from build123d import *

# Parameters (mm, degrees)
SKETCH1_W           = 20.32
SKETCH1_H           = 20.32
BOSS_EXTRUDE1_DEPTH = 1.905
CUT_EXTRUDE1_REACH  = 16.494
SKETCH2_R           = 1.2192
FILLET1_R           = 2.54


with BuildPart() as part:
    # Sketch1 → Boss-Extrude1 (new body)
    with BuildSketch(Plane.XY):
        Rectangle(SKETCH1_W, SKETCH1_H)
    extrude(amount=BOSS_EXTRUDE1_DEPTH)

    # Sketch2 → Cut-Extrude1 (cut, up to next)
    with BuildSketch(Plane.XY.offset(1.905), mode=Mode.PRIVATE) as cut_extrude1_sk1:
        with Locations((-7.62, 7.62)):
            Circle(SKETCH2_R)
    cut_extrude1_tool1 = extrude(cut_extrude1_sk1.sketch, amount=-CUT_EXTRUDE1_REACH, mode=Mode.PRIVATE) & part.part
    # Sketch2 → Cut-Extrude1 (cut, up to next)
    with BuildSketch(Plane.XY.offset(1.905), mode=Mode.PRIVATE) as cut_extrude1_sk2:
        with Locations((7.62, 7.62)):
            Circle(SKETCH2_R)
    cut_extrude1_tool2 = extrude(cut_extrude1_sk2.sketch, amount=-CUT_EXTRUDE1_REACH, mode=Mode.PRIVATE) & part.part
    add(cut_extrude1_tool1.solids().sort_by_distance((-7.62, 7.62, 1.905))[0], mode=Mode.SUBTRACT)
    add(cut_extrude1_tool2.solids().sort_by_distance((7.62, 7.62, 1.905))[0], mode=Mode.SUBTRACT)

    # Fillet1
    fillet1_edges = [part.edges().sort_by_distance(p)[0] for p in [
        (-10.16, 10.16, 0.9525),
        (10.16, 10.16, 0.9525),
        (10.16, -10.16, 0.9525),
        (-10.16, -10.16, 0.9525),
    ]]
    fillet(fillet1_edges, radius=FILLET1_R)


solid = part.part
Here's how the part is built. I have some questions about the finished solid (model axes, mm). Give positions to 0.01 mm unless a question says otherwise; leave off trailing zeros. Order: outer loops, then holes, each group sorted by start corner. A loop starts at its lowest first (then second) coordinate and runs counter-clockwise, first axis right, second up. Notation, with made-up numbers: (39.25, 15.5) -> (64.25, 15.5) arc R5 cw to (64.25, 24.5) -> close; hole circle Ø10 at (79, -39). An arc over 180 degrees is marked (long way). One line per item, written item: value. Start each with the question number.
1. Imagine slicing it at A-A, the plane z = 0.55. List the corners of the cut face in (x, y) for me.
2. We'd pull the mould along X, two halves only. Please class faces 1 (the face through (0, 10.16, 1)), 2 (the face through (9.396, -9.436, 0.966)), 3 (the face through (8.275, 8.648, 0.966)): released by +X, released by -X, zero draft, split by the parting line, or undercut.
3. I need wall thicknesses on probe 1 along Y at (x, z) = (-7.62, 0.75); probe 2 along Y at (x, z) = (8, 1.2); probe 3 along X at (y, z) = (-8.5, 1.5). Which ranges of each line are inside material? Lowest first, please. Write a range as from..to.
Values follow:
1. outline: (-10.16, -7.62) arc R2.54 ccw to (-7.62, -10.16) -> (7.62, -10.16) arc R2.54 ccw to (10.16, -7.62) -> (10.16, 7.62) arc R2.54 ccw to (7.62, 10.16) -> (-7.62, 10.16) arc R2.54 ccw to (-10.16, 7.62) -> close; hole circle Ø2.44 at (-7.62, 7.62); hole circle Ø2.44 at (7.62, 7.62)
2. face 1: zero draft
2. face 2: released by +X
2. face 3: undercut
3. probe 1: y = -10.16..6.4, 8.84..10.16
3. probe 2: y = -10.13..6.46, 8.78..10.13
3. probe 3: x = -10..10
